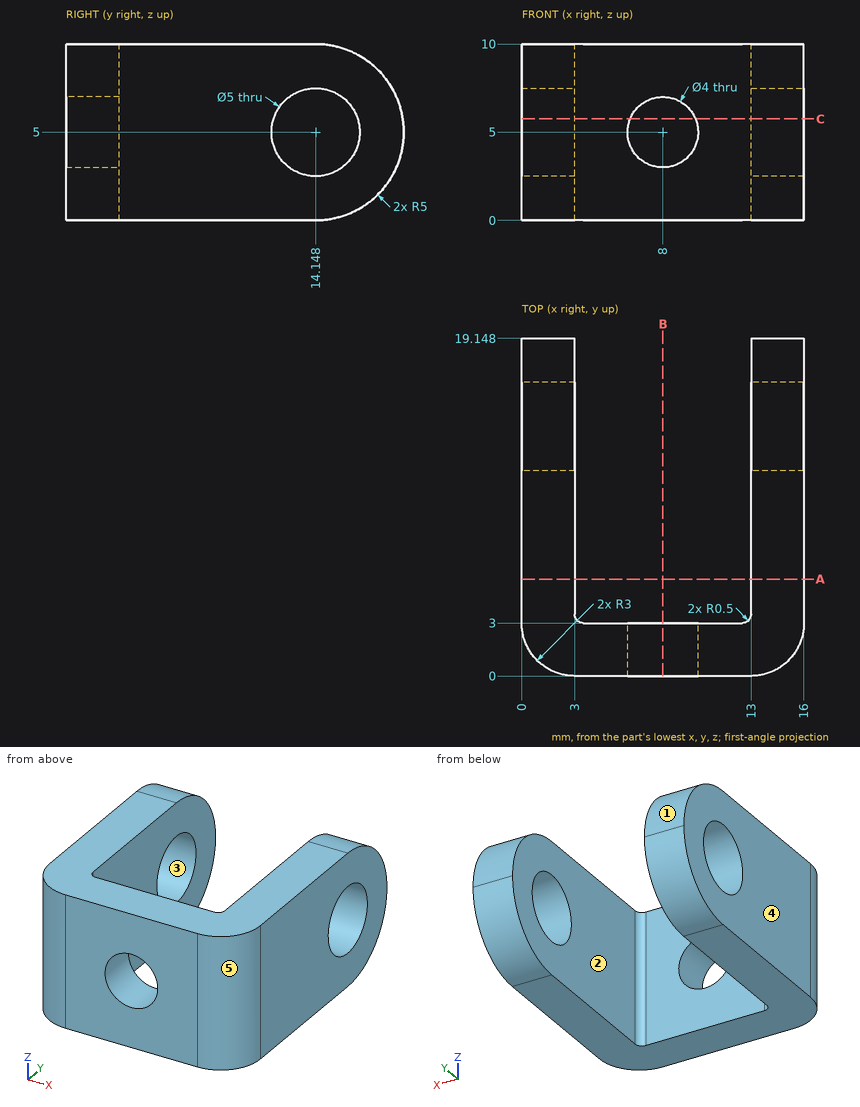
Design review of the part shown in the three views and the two pictorial views. Dimensions are in mm from the part's minimum x, y and z. A direction names the side the tool comes from. Coordinates: 2 decimals unless noted, no trailing zeros. Loops run counter-clockwise (first coordinate to the right, second up) from the corner with the lowest first, then second, coordinate; pieces in that order, holes last. Notation, with made-up numbers: M -24.75,-35.75 L 33.25,-35.75 A9 ccw 33.25,-19.75 Z; hole C 62.25,-17 d2. An arc over 180 degrees is marked long. Put each result on its own line as item: value. Start each with the question number.
Q1. For the marked faces 1 and 2, list the 3-axis set-ups (+Z, -Z, +X, -X, +Y, -Y) from which the entire face can be reached by the end or side of a thin tool; tool diameter is ignored.
Q2. Add section B-B (x = 8). Write out the cut boundary in (y, z).
Q3. Add section C-C (z = 5.75). Write out the cut boundary in (x, y).
Q4. The part is to be moulded in two halves that separate along Y. For the marked faces 3, 4 and 5, say which applies: +Y half, -Y half, draft (parallel to the pull), parting line (faces both ways), or undercut.
Q5. Clearance check with flat-ended pins moving along their axes: pin 1 (3 mm diameter, centred on x = 2.5, y = 17, fed in from +Z); pin 2 (5 mm diameter, centred on x = 5, z = 2, fed in from -Y); pin 3 (3.5 mm diameter, centred on x = 8, z = 5, fed in from -Y); pin 4 (4.5 mm diameter, centred on x = 8.5, z = 3, fed in from +Y). State where each tip first meets the part, or that it passes through.
Q6. Add section A-A (y = 5.5). Write out the cut boundary in (x, z), and give its area (3 significant figures).
Q7. Wall thickness on line 1 (X direction, y = 16.75, z = 6.25); line 2 (Y direction, x = 5, z = 6.5); line 3 (Y direction, x = 14, z = 5): over which ranges is each line inside the solid? List them lowest first.
Answers:
1. face 1: +Z, +X, -X, +Y
1. face 2: +Z, -Z, +Y
2. outline: M 0,0 L 3,0 L 3,3 L 0,3 Z; M 0,7 L 3,7 L 3,10 L 0,10 Z
3. outline: M 0,3 A3 ccw 3,0 L 6.15,0 L 6.15,3 L 3.5,3 A0.5 cw 3,3.5 L 3,11.76 L 0,11.76 Z; M 0,16.53 L 3,16.53 L 3,19.09 L 0,19.09 Z; M 9.85,0 L 13,0 A3 ccw 16,3 L 16,11.76 L 13,11.76 L 13,3.5 A0.5 cw 12.5,3 L 9.85,3 Z; M 13,16.53 L 16,16.53 L 16,19.09 L 13,19.09 Z
4. face 3: undercut
4. face 4: draft
4. face 5: -Y half
5. pin 1: stops at z = 9.81
5. pin 2: stops at y = 0
5. pin 3: passes through
5. pin 4: stops at y = 3
6. outline: M 0,0 L 3,0 L 3,10 L 0,10 Z; M 13,0 L 16,0 L 16,10 L 13,10 Z
6. area: 60.0 mm^2
7. line 1: x = 0 to 3, 13 to 16
7. line 2: y = 0 to 3
7. line 3: y = 0.17 to 11.65, 16.65 to 19.15
